The model under review builds one solid part; all positions refer to its coordinate system, in mm. A direction names the side the tool comes from. Give positions to 0.01 mm unless a question says otherwise; leave off trailing zeros. Order: outer loops, then holes, each group sorted by start corner. A loop starts at its lowest first (then second) coordinate and runs counter-clockwise, first axis right, second up. Notation, with made-up numbers: (9.25, 59) - (64.25, 59) arc R30 ccw to (64.25, 90) - close; hole circle Ø4 at (81.25, -27). An arc over 180 degrees is marked (long way). Answer as CSV lines item,"result". Start each with the question number.
from build123d import *

# Parameters (mm, degrees)
BOSS_EXTRUDE1_START     = -4.032483
SKETCH2_W               = 12.650748945
SKETCH2_H               = 65.169112304
BOSS_EXTRUDE1_DEPTH     = 12.7
BOSS_EXTRUDE3_START     = -4.032483117
BOSS_EXTRUDE3_OUTLINE_W = 12.650748945
BOSS_EXTRUDE3_OUTLINE_H = 7.62
BOSS_EXTRUDE3_DEPTH     = 15.24
SKETCH3_R               = 1.778
CUT_EXTRUDE1_DEPTH      = 7.62
SKETCH3_3_R             = 1.27
CUT_EXTRUDE2_DEPTH      = 68.330862042
CUT_EXTRUDE6_DEPTH      = 56.374578465
FILLET1_R               = 1.27
CAVITY1_START           = -22.170556152
CAVITY1_OUTLINE_W       = 12.650748945
CAVITY1_OUTLINE_H       = 5.08
CAVITY1_DEPTH           = 9.652


# Read off the part's stored shape, not the designer's step: Boss-Extrude3, Cavity1
with BuildPart() as part:
    # Sketch2 → Boss-Extrude1 (new body)
    with BuildSketch(Plane.XY.offset(BOSS_EXTRUDE1_START)):
        with Locations((27.23762425, -18.663141358)):
            Rectangle(SKETCH2_W, SKETCH2_H)
    extrude(amount=-BOSS_EXTRUDE1_DEPTH)

    # Boss-Extrude3 outline → Boss-Extrude3 (add)
    with BuildSketch(Plane.XY.offset(BOSS_EXTRUDE3_START)):
        with Locations((27.23762425, 10.111414794)):
            Rectangle(BOSS_EXTRUDE3_OUTLINE_W, BOSS_EXTRUDE3_OUTLINE_H)
        with BuildLine():
            Line((32.8, -5.914556152), (20.912249778, -5.914556152))
            Line((20.912249778, -5.914556152), (20.912249778, -31.798585206))
            Line((20.912249778, -31.798585206), (33.562998723, -31.798585206))
            Line((33.562998723, -31.798585206), (33.562998723, -6.065817947))
            ThreePointArc((33.562998723, -6.065817947), (33.188923894, -5.952736026), (32.8, -5.914556152))
        make_face()
        with Locations((27.23762425, -47.43769751)):
            Rectangle(BOSS_EXTRUDE3_OUTLINE_W, BOSS_EXTRUDE3_OUTLINE_H)
    extrude(amount=BOSS_EXTRUDE3_DEPTH)

    # Sketch3 → Cut-Extrude1 (cut)
    with BuildSketch(Plane(origin=(0, 0, -16.732483117), x_dir=(-1, 0, 0), z_dir=(0, 0, -1))):
        with Locations((-29.752998723, -18.663141358)):
            Circle(SKETCH3_R)
    extrude(amount=-CUT_EXTRUDE1_DEPTH, mode=Mode.SUBTRACT)

    # Sketch3<3> → Cut-Extrude2 (cut, through all)
    with BuildSketch(Plane(origin=(0, 0, -16.732483117), x_dir=(-1, 0, 0), z_dir=(0, 0, -1))):
        with Locations((-25.942998723, -12.313141358)):
            Circle(SKETCH3_3_R)
        with Locations((-25.942998723, -25.013141358)):
            Circle(SKETCH3_3_R)
    extrude(amount=-CUT_EXTRUDE2_DEPTH, mode=Mode.SUBTRACT)

    # Sketch7 → Cut-Extrude6 (cut, through all)
    with BuildSketch(Plane.ZY.offset(-20.912249778)):
        Polygon((11.207516883, 6.301414794), (11.207516883, 10.111414794), (-4.032483117, 6.301414794), align=None)
        Polygon((-4.032483117, -5.914556152), (11.207516883, -5.914556152), (11.207516883, -9.724556152), align=None)
        Polygon((-4.032483117, -43.62769751), (11.207516883, -47.43769751), (11.207516883, -43.62769751), align=None)
        Polygon((11.207516883, -31.798585206), (11.207516883, -27.988585206), (-4.032483117, -31.798585206), align=None)
    extrude(amount=-CUT_EXTRUDE6_DEPTH, mode=Mode.SUBTRACT)

    # Fillet1
    fillet1_edges = [part.edges().sort_by_distance(p)[0] for p in [
        (27.237624251, -9.724556152, 11.207516883),
        (27.23762425, -51.24769751, 11.207516883),
        (27.23762425, 13.921414794, 11.207516883),
        (27.237624251, 10.111414794, 11.207516883),
        (27.237624251, -27.988585206, 11.207516883),
        (27.237624251, -47.43769751, 11.207516883),
    ]]
    fillet(fillet1_edges, radius=FILLET1_R)

    # Cavity1 outline → Cavity1 (cut)
    with BuildSketch(Plane(origin=(0, 0, 0), x_dir=(1, 0, 0), z_dir=(0, 1, 0)).offset(CAVITY1_START)):
        with Locations((27.23762425, -6.762516883)):
            Rectangle(CAVITY1_OUTLINE_W, CAVITY1_OUTLINE_H)
    extrude(amount=CAVITY1_DEPTH, mode=Mode.SUBTRACT)


solid = part.part
Item 1: Mouldability with a two-part tool opening along Y and no side actions: class faces 4 (the face through (30, -19, -9.112)), 5 (the face through (27.326, 13.54, 10.845)), 6 (the face through (33.563, -19, -6)), 7 (the face through (28.8, -17.16, -12.98)) as released by +Y, released by -Y, zero draft, split by the parting line, or undercut.
Item 2: Take a section at A-A on z = 5. Write out the cut boundary in (x, y), and give its area (3 significant figures).
Item 3: Machinability: for faces 1 (the face through (27, 0, -4.032)), 2 (the face through (27, 13.921, -4)), 3 (the face through (27, -17, 9.303)), which of the approach directions +Z, -Z, +X, -X, +Y, -Y give a long, thin tool a straight path to every point of the face, cutting with its end or side? Answer none if there is none.
Item 4: Clearance check with a flat-ended pin moving along its axis: pin 1 (2 mm diameter, centred on x = 29.75, y = -18.66, fed in from -Z). State where the tip first meets the part, or that it passes through.
Item 5: For line 1 along Y through (x, z) = (26, 3.75); line 2 along Z through (x, y) = (23.75, -15.5); line 3 along Y through (x, z) = (23, 3.75), list the stretches that pass through material, from the lowest coordinate up.
Item 6: Take a section at D-D on y = -36. Write out the cut boundary in (x, z).
Item 7: Take a section at B-B on x = 23.5. Write out the cut boundary in (y, z).
Item 8: Take a section at C-C on z = -1.25. Write out the cut boundary in (x, y).
Data:
1,face 4,"undercut"
1,face 5,"released by +Y"
1,face 6,"zero draft"
1,face 7,"undercut"
2,outline,"(20.91, -51.25) - (33.56, -51.25) - (33.56, -45.89) - (20.91, -45.89) - close; (20.91, -29.54) - (33.56, -29.54) - (33.56, -22.17) - (20.91, -22.17) - close; (20.91, -12.52) - (24.69, -12.52) arc R1.27 cw (long way) to (27.2, -12.52) - (33.56, -12.52) - (33.56, -8.17) - (20.91, -8.17) - close; (20.91, 8.56) - (33.56, 8.56) - (33.56, 13.92) - (20.91, 13.92) - close; hole circle Ø2.54 at (25.94, -25.01)"
2,area,"276 mm^2"
3,face 1,"+Z, +X, -X"
3,face 2,"+Z, -Z, +X, -X, +Y"
3,face 3,"+X, -X"
4,pin 1,"stops at z = -9.11"
5,line 1,"y = -51.25 to -45.57, -29.85 to -26.28, -23.74 to -13.58, -11.04 to -7.86, 8.25 to 13.92"
5,line 2,"z = -16.73 to 4.22, 9.3 to 11.21"
5,line 3,"y = -51.25 to -45.57, -29.85 to -7.86, 8.25 to 13.92"
6,outline,"(20.91, -16.73) - (33.56, -16.73) - (33.56, -4.03) - (20.91, -4.03) - close"
7,outline,"(-51.25, -16.73) - (13.92, -16.73) - (13.92, 9.94) arc R1.27 ccw to (12.65, 11.21) - (11.1, 11.21) arc R1.27 ccw to (9.87, 10.25) - (6.3, -4.03) - (-5.91, -4.03) - (-9.48, 10.25) arc R1.27 ccw to (-10.72, 11.21) - (-27, 11.21) arc R1.27 ccw to (-28.23, 10.25) - (-31.8, -4.03) - (-43.63, -4.03) - (-47.2, 10.25) arc R1.27 ccw to (-48.43, 11.21) - (-49.98, 11.21) arc R1.27 ccw to (-51.25, 9.94) - close; hole (-22.17, 4.22) - (-12.52, 4.22) - (-12.52, 9.3) - (-22.17, 9.3) - close"
8,outline,"(20.91, -51.25) - (33.56, -51.25) - (33.56, -44.32) - (20.91, -44.32) - close; (20.91, -31.1) - (33.56, -31.1) - (33.56, -6.61) - (20.91, -6.61) - close; (20.91, 7) - (33.56, 7) - (33.56, 13.92) - (20.91, 13.92) - close; hole circle Ø2.54 at (25.94, -25.01); hole circle Ø2.54 at (25.94, -12.31)"
